Autodesk Inventor part; units mm, degrees
ref_plane "YZ Plane" through (0, 0, 0) normal (1, 0, 0) x (0, 1, 0)
ref_plane "XZ Plane" through (0, 0, 0) normal (0, 1, 0) x (-1, 0, 0)
ref_plane "XY Plane" through (0, 0, 0) normal (0, 0, 1) x (1, 0, 0)
sketch "スケッチ1" plane through (0, 0, 0) normal (0, 0, 1) x (1, 0, 0)
  circle A0 centre (0, 0) radius 2.5
  dimension "d0" = 5
extrude "押し出し1" add sketch "スケッチ1" along normal blind 20
sketch "スケッチ2" plane through (0, 0, 0) normal (0, 0, -1) x (-1, 0, 0)
  circle A0 centre (0, 0) radius 5
  dimension "d3" = 10
extrude "押し出し2" add sketch "スケッチ2" along normal blind 2.8
chamfer "面取り1" distance 2.5 angle 45 1 edges at (5, 0, 0)
sketch "スケッチ3" plane through (0, 0, -2.8) normal (0, 0, -1) x (-1, 0, 0)
  line L0 (0, 1.7321) -> (1.5, 0.866)
  line L1 (1.5, 0.866) -> (1.5, -0.866)
  line L2 (1.5, -0.866) -> (0, -1.7321)
  line L3 (0, -1.7321) -> (-1.5, -0.866)
  line L4 (-1.5, -0.866) -> (-1.5, 0.866)
  line L5 (-1.5, 0.866) -> (0, 1.7321)
  point P0 (0, 0)
  point P1 (0, 0)
  dimension "d12" = 3
extrude "押し出し3" cut sketch "スケッチ3" against normal blind 2.5
thread "ねじ1"
properties part number "M5皿ネジ 20" material "鉄 灰色"
CAD build for the part. Positions are in the model's coordinates, mm. A direction names the side the tool comes from. Coordinates: 2 decimals unless noted, no trailing zeros. Write each loop counter-clockwise with the first axis right and the second up, starting at its lowest first coordinate (ties: lowest second). Pieces come first, ordered by that corner, then holes.
(1) Drill centre lines: probe 1 along Z at (x, y) = (1.25, 0); probe 2 along X at (y, z) = (1.5, -1.5); probe 3 along X at (y, z) = (2, 14.5). Where is each one in solid material? Low to high.
(2) Flat gauge pins, fed straight in: pin 1 (2 mm diameter, centred on x = -4, y = 0, fed in from +Z); pin 2 (1.5 mm diameter, centred on y = 2, z = 6.5, fed in from -X); pin 3 (3 mm diameter, centred on x = -2, z = 14, fed in from -Y). Where does each tip first touch, or does it go through?
(3) Two-plate mould, pull along X, no slides. Class faces 1 (the face through (-0.54, 2.44, 9.86)), 2 (the face through (-0.76, -1.293, -1.568)), 3 (the face through (-2, 0, -2.8)): +X half, -X half, draft (parallel to the pull), parting line (faces both ways), or undercut.
(4) 3-axis set-ups, long thin cutter, end or side, ignore diameter. For faces 4 (the face through (-4.77, -1.5, -2.65)), 5 (the face through (0.76, 1.293, -1.568)): which of +Z, -Z, +X, -X, +Y, -Y reach the whole face in a straight line?
(5) Cut at B-B, the plane z = 12.5. List the corners of the cut face in (x, y).
Geometry says:
1. probe 1: z = -0.3 to 20
1. probe 2: x = -3.71 to -0.4, 0.4 to 3.71
1. probe 3: x = -1.5 to 1.5
2. pin 1: stops at z = -0.5
2. pin 2: stops at x = -2.17
2. pin 3: stops at y = -2.45
3. face 1: parting line
3. face 2: undercut
3. face 3: draft
4. face 4: +Z, -Z
4. face 5: -Z
5. outline: circle Ø5 at (0, 0)
